Job drawing, mm, ordinate dimensions from the low corner. One solid piece. Give positions to 0.01 mm unless a question says otherwise; leave off trailing zeros. One line per question, with ' | ' between items.
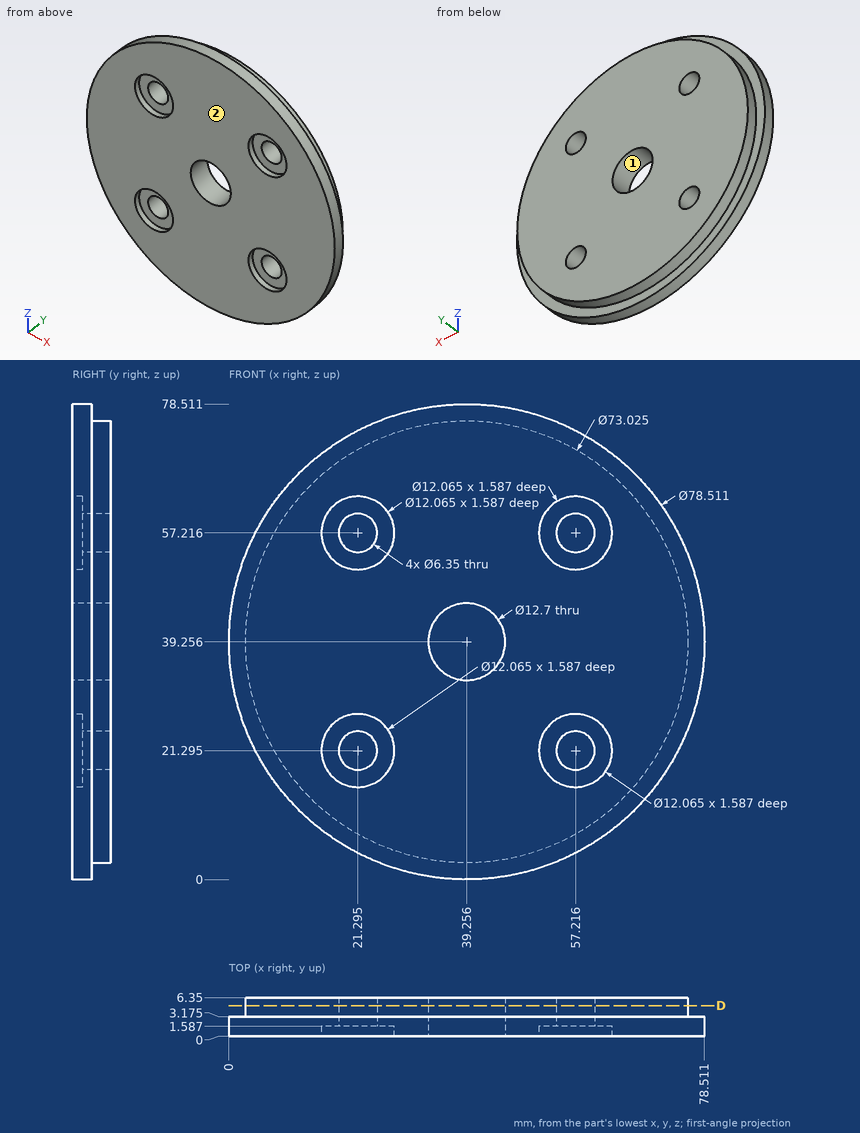
1. Probe L1, parallel to X at y = 1, z = 58 (1 decimal); L2, parallel to X at y = 1.25, z = 59 (1 decimal). List the from-to ranges inside material, lowest first. Write a range as from..to.
Worked out:
L1: x = 4.8..15.3, 27.3..51.2, 63.2..73.7 | L2: x = 5.3..15.5, 27.1..51.5, 63..73.2
2. Slice it at D-D on y = 5. Give the number of separate pieces and of enclosed holes in the cut face, then the cut area to 4 significant figures.
Worked out:
separate pieces: 1 | enclosed holes: 5 | area: 3,935 mm2
3. Drop flat-ended pins along their axis: pin 1 (6 mm diameter, centred on x = 58, z = 57, fed in from -Y); pin 2 (1 mm diameter, centred on y = 4.5, z = 52, fed in from +X) (1 decimal); pin 3 (1 mm diameter, centred on y = 3.5, z = 19.5, fed in from -X) (1 decimal). Give the stop position or say it passes through.
Worked out:
pin 1: stops at y = 1.59 | pin 2: stops at x = 73.7 | pin 3: stops at x = 5.1
4. Mould opens along X. For the marked faces 1 and 2 say: released by +X, released by -X, zero draft, split by the parting line, or undercut.
Worked out:
face 1: undercut | face 2: zero draft
